Autodesk Fusion 360 part; units mm, degrees
sketch "Sketch1" plane through (0, 0, 0) normal (0, 1, 0) x (1, 0, 0)
  line L0 (0, 0) -> (9.8, 0)
  line L1 (9.8, 0) -> (9.8, 14)
  line L2 (9.8, 14) -> (0, 14)
  line L3 (0, 14) -> (0, 0)
  line L4 (0, 9.6) -> (9.8, 9.6)
  dimension "d1" = 9.8
  dimension "d2" = 14
  dimension "d3" = 9.6
extrude "Extrude1" add sketch "Sketch1" along normal blind 0.6
extrude "Extrude2" add sketch "Sketch1" along normal blind 2.2 contours L0 L1 L3 L4
fillet "Fillet1" radius 0.9 4 edges at (4.9, 2.2, -9.6) (0, 2.2, -4.8) (4.9, 2.2, 0) (9.8, 2.2, -4.8)
The listing builds one solid part. Answer for the finished solid, in the listing's coordinates (mm). A direction names the side the tool comes from. Round coordinates to 2 decimals unless told otherwise and drop trailing zeros. Order: outer loops, then holes, each group sorted by start corner. A loop starts at its lowest first (then second) coordinate and runs counter-clockwise, first axis right, second up. Notation, with made-up numbers: (-32, 40) -> (10, 40) arc R16 cw to (10, 62) -> close; hole circle Ø6 at (79.25, 37.25). An arc over 180 degrees is marked (long way). Answer as CSV lines item,"result".
Q1. A cutting plane is placed at C-C on y = 0.95. Determine the outline of the cut face in (x, z).
Computed values:
outline,"(0, -9.6) -> (9.8, -9.6) -> (9.8, 0) -> (0, 0) -> close"
Q2. Consider line 1 (Z direction, x = 0.75, y = 0.8); line 2 (Y direction, x = 3.25, z = -10.75); line 3 (Z direction, x = 6.5, y = 2). Determine where each line is inside the solid, lowest interval first. Write a range as from..to.
Computed values:
line 1,"z = -9.6..0"
line 2,"y = 0..0.6"
line 3,"z = -9.27..-0.33"
Q3. Which of the six approach directions +Z, -Z, +X, -X, +Y, -Y give full straight-line access (tool end or side, diameter ignored) to faces 1 (the flat face through (5, 0.6, -12)), 2 (the cylindrical face through (4.97, 1.94, -0.27))?
Computed values:
face 1,"-Z, +X, -X, +Y"
face 2,"+Z, +X, -X, +Y"
Q4. A cutting plane is placed at D-D on z = -9.25. Determine the outline of the cut face in (x, y), plus the area to 3 significant figures.
Computed values:
outline,"(0, 0) -> (9.8, 0) -> (9.8, 1.3) arc R0.9 ccw to (9.45, 2.01) -> (0.35, 2.01) arc R0.9 ccw to (0, 1.3) -> close"
area,"19.6 mm^2"
Q5. A cutting plane is placed at B-B on z = -1.75. Determine the outline of the cut face in (x, y), plus the area to 3 significant figures.
Computed values:
outline,"(0, 0) -> (9.8, 0) -> (9.8, 1.3) arc R0.9 ccw to (8.9, 2.2) -> (0.9, 2.2) arc R0.9 ccw to (0, 1.3) -> close"
area,"21.2 mm^2"
Q6. Given pin 1 (2 mm diameter, centred on x = 3, z = -13, fed in from +Y), flat-ended and moving along its own axis, determine where the tip first touches the part or whether it passes through.
Computed values:
pin 1,"stops at y = 0.6"
Q7. A cutting plane is placed at A-A on x = 2. Determine the outline of the cut face in (y, z), plus the area to 3 significant figures.
Computed values:
outline,"(0, -14) -> (0.6, -14) -> (0.6, -9.6) -> (1.3, -9.6) arc R0.9 ccw to (2.2, -8.7) -> (2.2, -0.9) arc R0.9 ccw to (1.3, 0) -> (0, 0) -> close"
area,"23.4 mm^2"
